Verification items for the finished model (mm, model axes). A direction names the side the tool comes from. Give positions to 0.01 mm unless a question says otherwise; leave off trailing zeros. Write each loop counter-clockwise with the first axis right and the second up, starting at its lowest first coordinate (ties: lowest second). Pieces come first, ordered by that corner, then holes.
from build123d import *

# Parameters (mm, degrees)
F1_DEPTH = 50.8
F2_W     = 12.7
F2_H     = 12.7
F3_DEPTH = 50.801
F4_W     = 19.05
F4_H     = 25.4
F5_DEPTH = 50.801


with BuildPart() as f1:
    # F0 (on Front) → F1 (new body)
    with BuildSketch(Plane.XZ):
        Polygon((25.4, 50.8), (0, 50.8), (0, 0), (50.8, 0), (50.8, 31.212713), align=None)
    extrude(amount=F1_DEPTH)

    # F2 (on face) → F3 (cut, through all)
    with BuildSketch(Plane.XY.offset(50.8)):
        with Locations((6.35, -6.35)):
            Rectangle(F2_W, F2_H)
        with Locations((6.35, -44.45)):
            Rectangle(F2_W, F2_H)
    extrude(amount=-F3_DEPTH, mode=Mode.SUBTRACT)

    # F4 (on face) → F5 (cut, through all)
    with BuildSketch(Plane(origin=(0, 0, 0), x_dir=(1, 0, 0), z_dir=(0, 0, -1))):
        with Locations((41.275, 25.4)):
            Rectangle(F4_W, F4_H)
    extrude(amount=-F5_DEPTH, mode=Mode.SUBTRACT)


solid = f1.part
Item 1: Set-up check for faces 4 (the face through (41, -38.1, 18)), 5 (the face through (0, -25, 26)), 6 (the face through (6, -38.1, 26)), 7 (the face through (12.7, -6, 26)): record each of +Z, -Z, +X, -X, +Y, -Y from which the full face is reachable in a straight line by a thin tool's end or side.
Answer key:
face 4: +Z, -Z, +X
face 5: +Z, -Z, -X, +Y, -Y
face 6: +Z, -Z, -X, -Y
face 7: +Z, -Z, -X, +Y
Item 2: Depth check by flat-ended pin: pin 1 (1 mm diameter, centred on x = 6, y = -40, fed in from +Z); pin 2 (4 mm diameter, centred on x = 8.5, y = -30.5, fed in from -Z); pin 3 (4 mm diameter, centred on x = 4, z = 14.5, fed in from -Y); pin 4 (10 mm diameter, centred on x = 4.5, z = 30.5, fed in from +Y). Enter the tip coordinate at first touch or a pass-through.
Answer key:
pin 1: passes through
pin 2: stops at z = 0
pin 3: stops at y = -38.1
pin 4: stops at y = -12.7
Item 3: Sectioned sample at C-C on z = 32. Record the cut outline in (x, y).
Answer key:
outline: (0, -38.1) - (12.7, -38.1) - (12.7, -50.8) - (49.78, -50.8) - (49.78, -38.1) - (31.75, -38.1) - (31.75, -12.7) - (49.78, -12.7) - (49.78, 0) - (12.7, 0) - (12.7, -12.7) - (0, -12.7) - close
Item 4: Sectioned sample at A-A on x = 46.5. Record the cut outline in (y, z), then the cut area to 3 significant figures.
Answer key:
outline: (-50.8, 0) - (-38.1, 0) - (-38.1, 34.53) - (-50.8, 34.53) - close; (-12.7, 0) - (0, 0) - (0, 34.53) - (-12.7, 34.53) - close
area: 877 mm2
Item 5: Sectioned sample at B-B on y = -7. Record the cut outline in (x, z).
Answer key:
outline: (12.7, 0) - (50.8, 0) - (50.8, 31.21) - (25.4, 50.8) - (12.7, 50.8) - close
Item 6: Release check for a two-part mould opening along Y. For faces 1 (the face through (31, -50.8, 26)), 2 (the face through (25, -25, 0)), 3 (the face through (31.75, -25, 23)) record: released by +Y, released by -Y, zero draft, split by the parting line, or undercut.
Answer key:
face 1: released by -Y
face 2: zero draft
face 3: undercut
Item 7: Sectioned sample at D-D on y = -27.5. Record the cut outline in (x, z).
Answer key:
outline: (0, 0) - (31.75, 0) - (31.75, 45.9) - (25.4, 50.8) - (0, 50.8) - close
Item 8: Scan lines: line 1 along Y through (x, z) = (48.5, 19.5); line 2 along X through (y, z) = (-34.5, 42.5); line 3 along Y through (x, z) = (4, 15). Record each from-to range of solid material in increasing order.
Answer key:
line 1: y = -50.8 to -38.1, -12.7 to 0
line 2: x = 0 to 31.75
line 3: y = -38.1 to -12.7
